Verification items for the finished model (mm, model axes). A direction names the side the tool comes from. Round coordinates to 2 decimals unless told otherwise and drop trailing zeros. Write each loop counter-clockwise with the first axis right and the second up, starting at its lowest first coordinate (ties: lowest second). Pieces come first, ordered by that corner, then holes. Notation, with made-up numbers: (17, 18) - (24, 18) arc R26 ccw to (24, 34) - close; hole circle Ø5 at (85, 52.25). An arc over 180 degrees is marked (long way). Answer as a JSON object with one key per item and string values.
Autodesk Inventor part; units mm, degrees
ref_plane "YZ Plane" through (0, 0, 0) normal (1, 0, 0) x (0, 1, 0)
ref_plane "XZ Plane" through (0, 0, 0) normal (0, 1, 0) x (-1, 0, 0)
ref_plane "XY Plane" through (0, 0, 0) normal (0, 0, 1) x (1, 0, 0)
sketch "スケッチ1" plane through (0, 0, 0) normal (0, 0, 1) x (1, 0, 0)
  line L0 (-13.97, 24.13) -> (13.97, 24.13)
  line L1 (13.97, 24.13) -> (13.97, -24.13)
  line L2 (13.97, -24.13) -> (-13.97, -24.13)
  line L3 (-13.97, -24.13) -> (-13.97, 24.13)
  point P0 (0, 0)
  point P1 (-13.97, 0)
  point P2 (0, -24.13)
  dimension "d0" = 27.94
  dimension "d1" = 48.26
extrude "押し出し1" add sketch "スケッチ1" along normal blind 1.6
sketch "スケッチ2" plane through (0, 0, 0) normal (0, 0, -1) x (-1, 0, 0)
  line L0 (0, 28.1996) -> (0, -28.1996) construction
  line L1 (-12.7, -28.1996) -> (-12.7, 28.1996) construction
  line L2 (12.7, 28.1996) -> (12.7, -28.1996) construction
  line L3 (-11.43, 24.13) -> (-13.97, 24.13)
  line L4 (-13.97, 24.13) -> (-13.97, -24.13)
  line L5 (-13.97, -24.13) -> (-11.43, -24.13)
  line L6 (-11.43, -24.13) -> (-11.43, 24.13)
  line L7 (11.43, 24.13) -> (13.97, 24.13)
  line L8 (13.97, 24.13) -> (13.97, -24.13)
  line L9 (13.97, -24.13) -> (11.43, -24.13)
  line L10 (11.43, -24.13) -> (11.43, 24.13)
  line L11 (-13.97, -24.13) -> (-13.97, 24.13)
  line L12 (-13.97, 24.13) -> (13.97, 24.13)
  line L13 (13.97, 24.13) -> (13.97, -24.13)
  line L14 (13.97, -24.13) -> (-13.97, -24.13)
  point P0 (0, 0)
  point P1 (0, 0)
  point P2 (-12.7, 24.13)
  point P3 (12.7, 24.13)
  dimension "d4" = 25.4
  dimension "d5" = 2.54
extrude "押し出し2" add sketch "スケッチ2" along normal blind 11 contours L6 L5 L4 L3 | L7 L8 L9 L10
sketch "スケッチ3" plane through (0, 0, 1.6) normal (0, 0, 1) x (1, 0, 0)
  line L0 (-9, 30.13) -> (9, 30.13)
  line L1 (9, 30.13) -> (9, 5.13)
  line L2 (9, 5.13) -> (-9, 5.13)
  line L3 (-9, 5.13) -> (-9, 30.13)
  line L4 (13.97, 24.13) -> (-13.97, 24.13)
  point P0 (0, 0)
  point P1 (0, 5.13)
  dimension "d8" = 18
  dimension "d9" = 25
  dimension "d10" = 6
extrude "押し出し3" add sketch "スケッチ3" along normal blind 0.8
sketch "スケッチ4" plane through (0, 0, 2.4) normal (0, 0, 1) x (1, 0, 0)
  line L0 (-7.75, 23.63) -> (7.75, 23.63)
  line L1 (7.75, 23.63) -> (7.75, 6.63)
  line L2 (7.75, 6.63) -> (-7.75, 6.63)
  line L3 (-7.75, 6.63) -> (-7.75, 23.63)
  line L4 (-9, 5.13) -> (9, 5.13)
  point P0 (0, 0)
  point P1 (0, 6.63)
  dimension "d13" = 15.5
  dimension "d14" = 17
  dimension "d15" = 1.5
extrude "押し出し4" add sketch "スケッチ4" along normal blind 2.5
sketch "スケッチ5" plane through (0, 0, 1.6) normal (0, 0, 1) x (1, 0, 0)
  line L0 (-3.5, -18.63) -> (3.5, -18.63)
  line L1 (3.5, -18.63) -> (3.5, -25.63)
  line L2 (3.5, -25.63) -> (-3.5, -25.63)
  line L3 (-3.5, -25.63) -> (-3.5, -18.63)
  line L4 (-13.97, -24.13) -> (13.97, -24.13)
  point P0 (0, 0)
  point P1 (0, -18.63)
  dimension "d18" = 7
  dimension "d19" = 7
  dimension "d20" = 1.5
extrude "押し出し5" add sketch "スケッチ5" along normal blind 2.5
properties part number "ESP32-DevKitC"
Q1. Material ranges on line 1 along X through (y, z) = (16, -2); line 2 along Y through (x, z) = (1.75, 3.75); line 3 along Z through (x, y) = (11.25, 20), recorded low to high. Write a range as [from, to].
Geometry check:
{"line 1": "x = [-13.97, -11.43], [11.43, 13.97]", "line 2": "y = [-25.63, -18.63], [6.63, 23.63]", "line 3": "z = [0, 1.6]"}
Q2. Section check A-A, the plane z = -2.25. Record the cut outline in (x, y).
Geometry check:
{"outline": "(-13.97, -24.13) - (-11.43, -24.13) - (-11.43, 24.13) - (-13.97, 24.13) - close; (11.43, -24.13) - (13.97, -24.13) - (13.97, 24.13) - (11.43, 24.13) - close"}
Q3. Section check D-D, the plane x = 1.5. Record the cut outline in (y, z).
Geometry check:
{"outline": "(-25.63, 1.6) - (-24.13, 1.6) - (-24.13, 0) - (24.13, 0) - (24.13, 1.6) - (30.13, 1.6) - (30.13, 2.4) - (23.63, 2.4) - (23.63, 4.9) - (6.63, 4.9) - (6.63, 2.4) - (5.13, 2.4) - (5.13, 1.6) - (-18.63, 1.6) - (-18.63, 4.1) - (-25.63, 4.1) - close"}
Q4. Section check B-B, the plane y = 14. Record the cut outline in (x, z), then the cut area to 3 significant figures.
Geometry check:
{"outline": "(-13.97, -11) - (-11.43, -11) - (-11.43, 0) - (11.43, 0) - (11.43, -11) - (13.97, -11) - (13.97, 1.6) - (9, 1.6) - (9, 2.4) - (7.75, 2.4) - (7.75, 4.9) - (-7.75, 4.9) - (-7.75, 2.4) - (-9, 2.4) - (-9, 1.6) - (-13.97, 1.6) - close", "area": "154 mm2"}
Q5. Gauge pin test, flat ends, axial feed: P1, Ø8, axis at x = -8, z = -2, coming from the -Y side; P2, Ø8, axis at x = -3.5, y = 0, coming from the +Z side; P3, Ø5, axis at x = -3, y = 26.5, coming from the -Z side. Record the tip position at first contact, or that the pin passes through.
Geometry check:
{"P1": "stops at y = -24.13", "P2": "stops at z = 1.6", "P3": "stops at z = 0"}
Q6. Set-up check for faces 1 (the flat face through (-3.5, -22, 3)), 2 (the flat face through (0, 23.63, 4)), 3 (the flat face through (0, -22, 4.1)), 4 (the flat face through (0, 6.63, 4)): record each of +Z, -Z, +X, -X, +Y, -Y from which the full face is reachable in a straight line by a thin tool's end or side.
Geometry check:
{"face 1": "+Z, -X, -Y", "face 2": "+Z, +X, -X, +Y", "face 3": "+Z, +X, -X, -Y", "face 4": "+Z, +X, -X"}
Q7. Section check C-C, the plane x = 6. Record the cut outline in (y, z), then the cut area to 3 significant figures.
Geometry check:
{"outline": "(-24.13, 0) - (24.13, 0) - (24.13, 1.6) - (30.13, 1.6) - (30.13, 2.4) - (23.63, 2.4) - (23.63, 4.9) - (6.63, 4.9) - (6.63, 2.4) - (5.13, 2.4) - (5.13, 1.6) - (-24.13, 1.6) - close", "area": "140 mm2"}
